Check sheet for the modelled part. Datum: model origin and axes. Units: mm. Face numbers are marked on the shaded views. Round coordinates to 2 decimals unless told otherwise and drop trailing zeros. Write each loop counter-clockwise with the first axis right and the second up, starting at its lowest first coordinate (ties: lowest second). Pieces come first, ordered by that corner, then holes. Notation, with made-up numbers: (-19, -26) -> (6, -26) arc R22 cw to (6, -11) -> close; hole circle Ø9 at (22, 52.5). An arc over 180 degrees is marked (long way). Write item = value, one per line.
from build123d import *

# Parameters (mm, degrees)
BOSS_EXTRUDE1_DEPTH     = 16.668
CUT_EXTRUDE1_DEPTH      = 45.45
CUT_EXTRUDE1_DEPTH_BACK = 45.45
DRAFT1_ANGLE            = 1
CUT_EXTRUDE2_REACH      = 38.469
SKETCH3_R               = 5.5
CUT_EXTRUDE3_DEPTH      = 10
CUT_EXTRUDE4_REACH      = 38.469
SKETCH5_R               = 5.5
FILLET1_R               = 3


with BuildPart() as part:
    # Sketch1 → Boss-Extrude1 (new body, symmetric)
    with BuildSketch(Plane(origin=(0, 0, 0), x_dir=(0, 0, -1), z_dir=(1, 0, 0))):
        with BuildLine():
            Line((22.225, 38.494829198), (45.45, 25.085869196))
            Line((45.45, 25.085869196), (45.45, -25.085869196))
            Line((45.45, -25.085869196), (22.225, -38.494829198))
            ThreePointArc((22.225, -38.494829198), (-44.45, 0), (22.225, 38.494829198))
        make_face()
    extrude(amount=BOSS_EXTRUDE1_DEPTH, both=True)

    # Sketch2 → Cut-Extrude1 (cut, two sides)
    with BuildSketch(Plane(origin=(0, 0, 0), x_dir=(1, 0, 0), z_dir=(0, 1, 0))) as cut_extrude1_sk:
        with BuildLine():
            Line((-7.588316422, 21.130183578), (-0.129046134, 13.670913289))
            Line((-0.129046134, 13.670913289), (-1.143550449, -44.45))
            Line((-1.143550449, -44.45), (1.143550449, -44.45))
            Line((1.143550449, -44.45), (0.129046134, 13.670913289))
            Line((0.129046134, 13.670913289), (7.588316422, 21.130183578))
            ThreePointArc((7.588316422, 21.130183578), (0, 39.45), (-7.588316422, 21.130183578))
        make_face()
    extrude(amount=CUT_EXTRUDE1_DEPTH, mode=Mode.SUBTRACT)
    extrude(cut_extrude1_sk.sketch, amount=-CUT_EXTRUDE1_DEPTH_BACK, mode=Mode.SUBTRACT)

    # Draft1
    draft1_faces = [part.faces().sort_by_distance(p)[0] for p in [
        (16.668, 0, -1.658648034),
        (-16.668, 0, -1.658648034),
    ]]
    draft(draft1_faces, Plane(origin=(16.668, 25.085869196, -45.45), x_dir=(-1, 0, 0), z_dir=(0, 0, -1)), DRAFT1_ANGLE)

    # Sketch3 → Cut-Extrude2 (cut, up to next)
    with BuildSketch(Plane(origin=(17.456014215, 0, -0.304695862), x_dir=(-0.017452406, 0, -0.999847695), z_dir=(0.999847695, 0, -0.017452406)), mode=Mode.PRIVATE) as cut_extrude2_sk1:
        with Locations((-0.304742275, 0)):
            Circle(SKETCH3_R)
    cut_extrude2_tool1 = extrude(cut_extrude2_sk1.sketch, amount=-CUT_EXTRUDE2_REACH, mode=Mode.PRIVATE) & part.part
    add(cut_extrude2_tool1.solids().sort_by_distance((17.461333, 0, 0))[0], mode=Mode.SUBTRACT)

    # Sketch4 → Cut-Extrude3 (cut)
    with BuildSketch(Plane(origin=(17.456014215, 0, -0.304695862), x_dir=(-0.017452406, 0, -0.999847695), z_dir=(0.999847695, 0, -0.017452406))):
        Polygon((9.394742247, 0), (4.544999986, 8.4), (-5.154484536, 8.4), (-10.004226798, 0), (-5.154484536, -8.4), (4.544999986, -8.4), align=None)
    extrude(amount=-CUT_EXTRUDE3_DEPTH, mode=Mode.SUBTRACT)

    # Sketch5 → Cut-Extrude4 (cut, up to next)
    with BuildSketch(Plane(origin=(-17.456014215, 0, -0.304695862), x_dir=(-0.017452406, 0, 0.999847695), z_dir=(-0.999847695, 0, -0.017452406)), mode=Mode.PRIVATE) as cut_extrude4_sk1:
        with Locations((0.304742275, 0)):
            Circle(SKETCH5_R)
    cut_extrude4_tool1 = extrude(cut_extrude4_sk1.sketch, amount=-CUT_EXTRUDE4_REACH, mode=Mode.PRIVATE) & part.part
    add(cut_extrude4_tool1.solids().sort_by_distance((-17.461333, 0, 0))[0], mode=Mode.SUBTRACT)

    # Fillet1
    fillet1_edges = [part.edges().sort_by_distance(p)[0] for p in [
        (16.870696941, 31.790349197, -33.8375),
        (18.237210337, 0.000220739, 44.449999999),
        (-16.870696941, 31.790349197, -33.8375),
        (-16.870697084, -31.790353899, -33.837491856),
        (-18.237210337, 9.404e-06, 44.45),
        (16.870700278, -31.790459554, -33.837308856),
    ]]
    fillet(fillet1_edges, radius=FILLET1_R)


solid = part.part
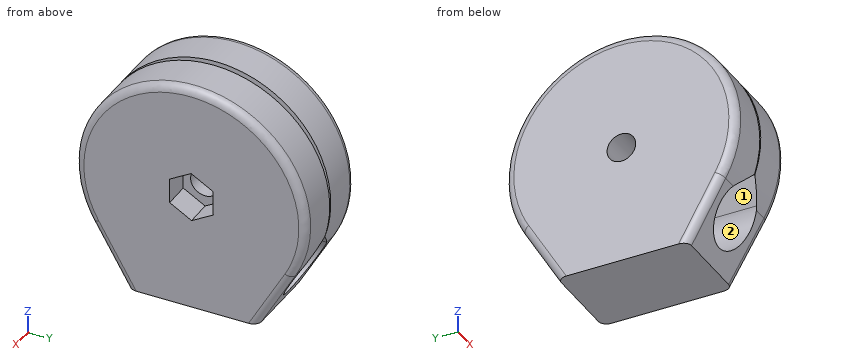
(1) Material ranges on L1, parallel to Z at x = 0, y = 16; L2, parallel to Z at x = 6, y = -20.5; L3, parallel to X at y = 17, z = 35.5, recorded low to high. Write a range as [from, to].
Worked answers:
L1 = [-45.45, -39.45]
L2 = [-45.45, -37.62], [-19.54, 39.44]
L3 = [-18.08, -0.99], [0.99, 18.08]
(2) Sectioned sample at B-B on z = 0. Count the separate pieces of the cut face and the enclosed holes in it, then the cut area to 3 significant figures.
Worked answers:
separate_pieces = 4
enclosed_holes = 0
area = 2,600 mm²
(3) Go/stop test with flat-tipped pins: P1, Ø1, axis at y = -3.5, z = -21, coming from the +X side; P2, Ø3, axis at x = 5, z = -10.5, coming from the -Y side; P3, Ø6, axis at x = -7.5, y = 3.5, coming from the +Z side. Record where each tip stops, or that it passes through.
Worked answers:
P1 = 17.1
P2 = -43.53
P3 = 44.45
(4) Sectioned sample at A-A on x = 12.5. Enter the section's corners in (y, z) (3 decimals), then the cut area to 3 significant figures.
Worked answers:
outline = (-38.495, -22.225) -> (-25.086, -45.45) -> (25.086, -45.45) -> (38.495, -22.225) arc R44.45 ccw (long way) to start; hole (-8.4, -4.764) -> (0, -9.614) -> (8.4, -4.764) -> (8.4, 4.937) -> (0, 9.788) -> (-8.4, 4.937) -> close
area = 6,230 mm²
(5) Release check for a two-part mould opening along X. For the marked faces 1 and 2 record: pulls with the +X half, pulls with the -X half, needs draft (parallel to the pull), parting line crosses it, or undercut.
Worked answers:
face_1 = undercut
face_2 = undercut
